The figure shows three views and two pictorial views of one solid part (mm, origin at its lowest corner). Answer the questions. Round coordinates to 2 decimals unless told otherwise and drop trailing zeros. Order: outer loops, then holes, each group sorted by start corner. A loop starts at its lowest first (then second) coordinate and runs counter-clockwise, first axis right, second up. Notation, with made-up numbers: (-22.75, -9) -> (17.25, -9) arc R25 cw to (17.25, 3) -> close; hole circle Ø8 at (70.25, 82). An arc over 180 degrees is marked (long way). Answer as a JSON object with one key per item and string values. Group by question number.
Item 1: Section B-B, the plane x = 54 is taken. Write down the section's boundary in (y, z).
Item 2: Given P1, Ø1.5, axis at y = 8, z = 54.5, coming from the -X side (1 decimal); P2, Ø6, axis at x = 17.5, y = 6.5, coming from the +Z side; P3, Ø9, axis at x = 54, z = 12, coming from the +Y side; P4, Ø1, axis at y = 10.5, z = 67.5, coming from the -X side (1 decimal), each flat-ended and moving along its own axis, determine where each tip first touches the part or whether it passes through.
Item 3: The mould has two halves that part along X. Classify the marked faces 1, 2, 3 and 4: pulls with the +X half, pulls with the -X half, needs draft (parallel to the pull), parting line crosses it, or undercut.
Item 4: Section C-C, the plane z = 72.5 is taken. Write down the section's boundary in (x, y) (1 decimal).
Item 5: Section A-A, the plane y = 1 is taken. Count the separate pieces of the cut face and the enclosed holes in it, plus the area to 3 significant figures.
Item 6: Consider probe 1 along Z at (x, y) = (46.5, 1.5) (1 decimal); probe 2 along X at (y, z) = (1.5, 71.5) (1 decimal); probe 3 along X at (y, z) = (7.5, 46). Determine where each line is inside the solid, lowest interval first. Write a range as from..to.
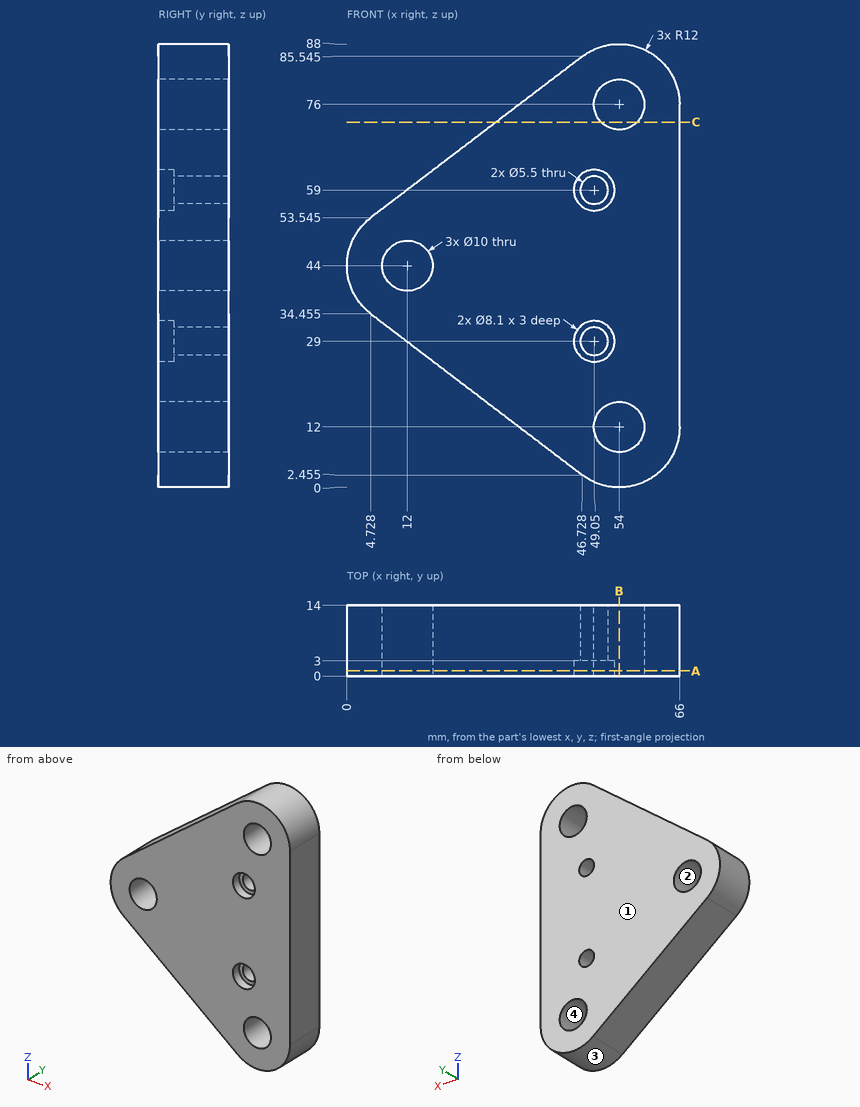
Values found:
{
 "1": {"outline": "(0, 0) -> (14, 0) -> (14, 7) -> (0, 7) -> close; (0, 17) -> (14, 17) -> (14, 71) -> (0, 71) -> close; (0, 81) -> (14, 81) -> (14, 88) -> (0, 88) -> close"},
 "2": {"P1": "x = 5", "P2": "z = 65.56", "P3": "through", "P4": "x = 22.4"},
 "3": {"face 1": "needs draft", "face 2": "undercut", "face 3": "parting line crosses it", "face 4": "undercut"},
 "4": {"outline": "(29.6, 0) -> (50.4, 0) -> (50.4, 14) -> (29.6, 14) -> close; (57.6, 0) -> (66, 0) -> (66, 14) -> (57.6, 14) -> close"},
 "5": {"separate pieces": "1", "enclosed holes": "5", "area": "3,490 mm2"},
 "6": {"probe 1": "2.6..25.9, 32.1..55.9, 62.1..85.4", "probe 2": "28.3..51.8, 56.2..66", "probe 3": "0.17..7.42, 16.58..66"}
}
